Part model, mm, in its own coordinate system. Give positions to 0.01 mm unless a question says otherwise; leave off trailing zeros. Write each loop counter-clockwise with the first axis right and the second up, starting at its lowest first coordinate (ties: lowest second). Pieces come first, ordered by that corner, then holes. Notation, with made-up numbers: M 32,1 L 84,1 A20 cw 84,13 Z; hole C 12.25,63 d11. An arc over 180 degrees is marked long. Answer as CSV lines item,"result". Start each with the question number.
1) Mould opens along X. For faces 1 (the cylindrical face through (-62.114, 10.406, 0.493)), 2 (the flat face through (11.92, 16.42, 0.99)), 3 (the cylindrical face through (8.53, 11.2, 0.49)), 4 (the flat face through (-63.32, 4.28, 0.99)) say: pulls with the +X half, pulls with the -X half, needs draft (parallel to the pull), parting line crosses it, or undercut.
2) Pin check, flat tip, straight feed: pin 1 Ø1.5 at (x, y) = (9.45, 10.35) entering from +Z. Stop position of the tip, or through.
3) Slice it at B-B, the plane y = 4.5. Give the cut face in (x, z).
4) Slice it at A-A, the plane y = 16.75. Give the cut face in (x, z), plus the area to 3 significant figures.
5) Wall check: line 1 along X through (y, z) = (9.25, 0.5); line 2 along X through (y, z) = (11, 1.7); line 3 along X through (y, z) = (15.75, 1.05). Give the ranges that are in metal, low to high. Write a range as from..to.
```python
from build123d import *

# Parameters (mm, degrees)
SKETCH_1_R      = 1.254908563
EXTRUDE_1_DEPTH = 2
CHAMFER_1_SIZE  = 1
CHAMFER_3_SIZE  = 0.5
CHAMFER_4_SIZE  = 0.5


with BuildPart() as part:
    # 草图1 → 凸台-拉伸1 (new body)
    with BuildSketch(Plane.XY):
        Polygon((-65.859878879, 17.884443478), (-64.859878879, 18.884443478), (9.454269131, 18.884443478), (14.454269131, 13.884443478), (14.454269131, 2.817687026), (13.454269131, 1.817687026), (-60.859878879, 1.817687026), (-65.859878879, 6.817687026), align=None)
        with Locations((-60.859878879, 10.351065252)):
            Circle(SKETCH_1_R, mode=Mode.SUBTRACT)
        with Locations((9.454269131, 10.351065252)):
            Circle(SKETCH_1_R, mode=Mode.SUBTRACT)
    extrude(amount=EXTRUDE_1_DEPTH)

    # 倒角1
    chamfer_1_edges = [part.edges().sort_by_distance(p)[0] for p in [
        (-62.114787442, 10.351065252, 2),
        (8.199360568, 10.351065252, 2),
    ]]
    chamfer(chamfer_1_edges, length=CHAMFER_1_SIZE)

    # 倒角3
    chamfer_3_edges = [part.edges().sort_by_distance(p)[0] for p in [
        (-65.859878879, 12.351065252, 2),
        (-63.359878879, 4.317687026, 2),
        (-23.702804874, 1.817687026, 2),
        (13.954269131, 2.317687026, 2),
        (14.454269131, 8.351065252, 2),
        (11.954269131, 16.384443478, 2),
        (-27.702804874, 18.884443478, 2),
        (-65.359878879, 18.384443478, 2),
    ]]
    chamfer(chamfer_3_edges, length=CHAMFER_3_SIZE)

    # 倒角4
    chamfer_4_edges = [part.edges().sort_by_distance(p)[0] for p in [
        (-65.359878879, 18.384443478, 0),
        (-27.702804874, 18.884443478, 0),
        (11.954269131, 16.384443478, 0),
        (14.454269131, 8.351065252, 0),
        (13.954269131, 2.317687026, 0),
        (-23.702804874, 1.817687026, 0),
        (-63.359878879, 4.317687026, 0),
        (-65.859878879, 12.351065252, 0),
    ]]
    chamfer(chamfer_4_edges, length=CHAMFER_4_SIZE)


solid = part.part
```
Found:
1,face 1,"undercut"
1,face 2,"pulls with the +X half"
1,face 3,"undercut"
1,face 4,"pulls with the -X half"
2,pin 1,"through"
3,outline,"M -63.54,0.5 L -62.84,0 L 13.95,0 L 14.45,0.5 L 14.45,1.5 L 13.95,2 L -62.84,2 L -63.54,1.5 Z"
4,outline,"M -65.86,0.5 L -65.36,0 L 10.88,0 L 11.59,0.5 L 11.59,1.5 L 10.88,2 L -65.36,2 L -65.86,1.5 Z"
4,area,"154 mm²"
5,line 1,"-65.86..-61.46, -60.26..8.85, 10.06..14.45"
5,line 2,"-65.66..-62.7, -59.02..7.61, 11.3..14.25"
5,line 3,"-65.86..12.59"
